Input: part model. Units: mm. Frame: model coordinates. A direction names the side the tool comes from. Give positions to 0.01 mm unless a question says otherwise; leave off trailing zeros. Loops run counter-clockwise (first coordinate to the right, second up) from the corner with the lowest first, then second, coordinate; pieces in that order, holes last. Notation, with made-up numbers: (-14, -14) -> (-7, -14) arc R25 cw to (-7, 22) -> close; hole circle Ø1 at (7.5, -21). An arc over 180 degrees is marked (long way). Use CSV: the item, a comma, the result in double quotes.
Autodesk Inventor part; units mm, degrees
ref_plane "YZ Plane" through (0, 0, 0) normal (1, 0, 0) x (0, 1, 0)
ref_plane "XZ Plane" through (0, 0, 0) normal (0, 1, 0) x (-1, 0, 0)
ref_plane "XY Plane" through (0, 0, 0) normal (0, 0, 1) x (1, 0, 0)
sketch "Sketch3" plane through (0, 0, 0) normal (0, 1, 0) x (-1, 0, 0)
  line L0 (0, 0) -> (0, -47) construction
  line L1 (-14.5, 0) -> (-14.5, -47)
  line L2 (14.5, -47) -> (14.5, 0)
  arc A0 (14.5, 0) -> (-14.5, 0) centre (0, 0) ccw
  arc A1 (-14.5, -47) -> (14.5, -47) centre (0, -47) ccw
  line L3 (0, 0) -> (47, 0) construction
  circle A2 centre (0, 0) radius 4.375
  circle A3 centre (0, -47) radius 4.375
  point P0 (0, -23.5)
  dimension "d8" = 47
  dimension "d9" = 90
  dimension "d10" = 29
  dimension "d11" = 8.75
  dimension "d12" = 8.75
extrude "Extrusion3" add sketch "Sketch3" along normal blind 2
sketch "Sketch4" plane through (0, 2, 0) normal (0, 1, 0) x (1, 0, 0)
  circle A0 centre (0, 0) radius 4.375
  circle A1 centre (0, 0) radius 2.75
  circle A2 centre (0, 47) radius 4.375
  circle A3 centre (0, 47) radius 2.75
  circle A4 centre (0, 0) radius 6
  circle A5 centre (0, 47) radius 6
  dimension "d15" = 12
  dimension "d16" = 12
extrude "Extrusion4" add sketch "Sketch4" along normal blind 3 contours A4 | A5
properties part number "Belt_Washer"
1) Contact query for flat-ended pins moving along their axis: pin 1 (3 mm diameter, centred on x = -9, y = 0.5, fed in from +Z); pin 2 (1 mm diameter, centred on x = -8, z = -51, fed in from +Y). Output: stop coordinate, or through.
From the geometry:
pin 1,"stops at z = 12.41"
pin 2,"stops at y = 2"
2) Reachability of faces 1 (the flat face through (-3, 5, 4)), 2 (the cylindrical face through (-1.301, 3.479, -52.857)) from +Z, -Z, +X, -X, +Y, -Y: full face, straight path, thin tool, end or side. Return the list, or none.
From the geometry:
face 1,"+Z, -Z, +X, -X, +Y"
face 2,"+Y"
3) Section query C-C (z = -30). Return loops of the section in (x, y), then the cut area to 3 significant figures.
From the geometry:
outline,"(-14.5, 0) -> (14.5, 0) -> (14.5, 2) -> (-14.5, 2) -> close"
area,"58.0 mm^2"
4) Mould query, pull axis Z, two halves, no side actions, for faces 3 (the flat face through (-3, 5, -43)), 4 (the cylindrical face through (-6, 3, 0)), 5 (the flat face through (0, 2, -23)), 6 (the cylindrical face through (-0.319, 0.986, -61.496)). Classes: pulls with the +Z half, pulls with the -Z half, needs draft (parallel to the pull), parting line crosses it, or undercut.
From the geometry:
face 3,"needs draft"
face 4,"undercut"
face 5,"undercut"
face 6,"pulls with the -Z half"
5) Ray query, line 1 (Z direction, x = 0, y = 1.25) (3 decimals); line 2 (Z direction, x = 0, y = 3.5) (3 decimals); line 3 (X direction, y = 3.9, z = 0) (3 decimals). Return the intervals inside material, ascending.
From the geometry:
line 1,"z = -61.5 to -51.375, -42.625 to -4.375, 4.375 to 14.5"
line 2,"z = -53 to -51.375, -42.625 to -41, -6 to -4.375, 4.375 to 6"
line 3,"x = -6 to -4.375, 4.375 to 6"
6) Section query A-A (y = 3.1). Return loops of the section in (x, z) (3 decimals).
From the geometry:
outline,"circle Ø12 at (0, -47); circle Ø12 at (0, 0); hole circle Ø8.75 at (0, -47); hole circle Ø8.75 at (0, 0)"
